from build123d import *

# Parameters (mm, degrees)
SALIENTE_EXTRUIR1_DEPTH = 1.6
CROQUIS3_R              = 4.2
SALIENTE_EXTRUIR2_DEPTH = 3
CROQUIS4_R              = 4.6
CORTAR_EXTRUIR1_DEPTH   = 1
CROQUIS5_R              = 3.5
CROQUIS5_R_2            = 3.45
SALIENTE_EXTRUIR3_DEPTH = 1
CROQUIS6_R              = 0.875
CORTAR_EXTRUIR2_DEPTH   = 22.438435028
CROQUIS7_R              = 1.4
CORTAR_EXTRUIR3_DEPTH   = 22.246329011
CROQUIS8_R              = 2.65
CORTAR_EXTRUIR4_DEPTH   = 3.4


with BuildPart() as part:
    # Croquis1 → Saliente-Extruir1 (new body)
    with BuildSketch(Plane(origin=(0, 0, 0), x_dir=(1, 0, 0), z_dir=(0, 1, 0))):
        with BuildLine():
            ThreePointArc((2.35, 13.321654392), (0, 15.671654392), (-2.35, 13.321654392))
            Line((-2.35, 13.321654392), (-3.5, 6.062177826))
            Line((-3.5, 6.062177826), (-10.361891124, 8.695986895))
            ThreePointArc((-10.361891124, 8.695986895), (-13.572050822, 7.835827196), (-12.711891124, 4.625667497))
            Line((-12.711891124, 4.625667497), (-7, 0))
            Line((-7, 0), (-12.711891124, -4.625667497))
            ThreePointArc((-12.711891124, -4.625667497), (-13.572050822, -7.835827196), (-10.361891124, -8.695986895))
            Line((-10.361891124, -8.695986895), (-3.5, -6.062177826))
            Line((-3.5, -6.062177826), (-2.35, -13.321654392))
            ThreePointArc((-2.35, -13.321654392), (0, -15.671654392), (2.35, -13.321654392))
            Line((2.35, -13.321654392), (3.5, -6.062177826))
            Line((3.5, -6.062177826), (10.361891124, -8.695986895))
            ThreePointArc((10.361891124, -8.695986895), (13.572050822, -7.835827196), (12.711891124, -4.625667497))
            Line((12.711891124, -4.625667497), (7, 0))
            Line((7, 0), (12.711891124, 4.625667497))
            ThreePointArc((12.711891124, 4.625667497), (13.572050822, 7.835827196), (10.361891124, 8.695986895))
            Line((10.361891124, 8.695986895), (3.5, 6.062177826))
            Line((3.5, 6.062177826), (2.35, 13.321654392))
        make_face()
    extrude(amount=SALIENTE_EXTRUIR1_DEPTH)

    # Croquis3 → Saliente-Extruir2 (add)
    with BuildSketch(Plane.XZ):
        with Locations(Location((0, 0, 0), (0, 0, 90))):
            Circle(CROQUIS3_R)
    extrude(amount=SALIENTE_EXTRUIR2_DEPTH)

    # Croquis4 → Cortar-Extruir1 (cut)
    with BuildSketch(Plane(origin=(0, 1.6, 0), x_dir=(1, 0, 0), z_dir=(0, 1, 0))):
        with Locations(Location((0, 0, 0), (0, 0, 270))):
            Circle(CROQUIS4_R)
    extrude(amount=-CORTAR_EXTRUIR1_DEPTH, mode=Mode.SUBTRACT)

    # Croquis5 → Saliente-Extruir3 (add)
    with BuildSketch(Plane(origin=(0, 0.6, 0), x_dir=(1, 0, 0), z_dir=(0, 1, 0))):
        with Locations(Location((0, 0, 0), (0, 0, 270))):
            Circle(CROQUIS5_R)
        with Locations(Location((0, 0, 0), (0, 0, 270))):
            Circle(CROQUIS5_R_2, mode=Mode.SUBTRACT)
    extrude(amount=SALIENTE_EXTRUIR3_DEPTH)

    # Croquis6 → Cortar-Extruir2 (cut, through all)
    with BuildSketch(Plane(origin=(0, 1.6, 0), x_dir=(1, 0, 0), z_dir=(0, 1, 0))):
        with Locations(Location((11.366583425, 6.5625, 0), (0, 0, 270))):
            Circle(CROQUIS6_R)
        with Locations(Location((9.114917375, 5.2625, 0), (0, 0, 270))):
            Circle(CROQUIS6_R)
        with Locations(Location((6.473539893, 3.7375, 0), (0, 0, 270))):
            Circle(CROQUIS6_R)
        with Locations(Location((11.366583425, -6.5625, 0), (0, 0, 270))):
            Circle(CROQUIS6_R)
        with Locations(Location((9.114917375, -5.2625, 0), (0, 0, 270))):
            Circle(CROQUIS6_R)
        with Locations(Location((6.473539893, -3.7375, 0), (0, 0, 270))):
            Circle(CROQUIS6_R)
        with Locations(Location((0, -13.125, 0), (0, 0, 270))):
            Circle(CROQUIS6_R)
        with Locations(Location((0, -10.525, 0), (0, 0, 270))):
            Circle(CROQUIS6_R)
        with Locations(Location((0, -7.475, 0), (0, 0, 270))):
            Circle(CROQUIS6_R)
        with Locations(Location((-11.366583425, -6.5625, 0), (0, 0, 270))):
            Circle(CROQUIS6_R)
        with Locations(Location((-9.114917375, -5.2625, 0), (0, 0, 270))):
            Circle(CROQUIS6_R)
        with Locations(Location((-6.473539893, -3.7375, 0), (0, 0, 270))):
            Circle(CROQUIS6_R)
        with Locations(Location((-11.366583425, 6.5625, 0), (0, 0, 270))):
            Circle(CROQUIS6_R)
        with Locations(Location((-9.114917375, 5.2625, 0), (0, 0, 270))):
            Circle(CROQUIS6_R)
        with Locations(Location((-6.473539893, 3.7375, 0), (0, 0, 270))):
            Circle(CROQUIS6_R)
        with Locations(Location((0, 13.125, 0), (0, 0, 270))):
            Circle(CROQUIS6_R)
        with Locations(Location((0, 10.525, 0), (0, 0, 270))):
            Circle(CROQUIS6_R)
        with Locations(Location((0, 7.475, 0), (0, 0, 270))):
            Circle(CROQUIS6_R)
    extrude(amount=-CORTAR_EXTRUIR2_DEPTH, mode=Mode.SUBTRACT)

    # Croquis7 → Cortar-Extruir3 (cut, through all)
    with BuildSketch(Plane(origin=(0, 0.6, 0), x_dir=(1, 0, 0), z_dir=(0, 1, 0))):
        with Locations(Location((0, 0, 0), (0, 0, 270))):
            Circle(CROQUIS7_R)
    extrude(amount=-CORTAR_EXTRUIR3_DEPTH, mode=Mode.SUBTRACT)

    # Croquis8 → Cortar-Extruir4 (cut)
    with BuildSketch(Plane.XZ.offset(3)):
        with Locations(Location((0, 0, 0), (0, 0, 270))):
            Circle(CROQUIS8_R)
    extrude(amount=-CORTAR_EXTRUIR4_DEPTH, mode=Mode.SUBTRACT)


solid = part.part
Source: CAD feature listing. Evaluate the final solid. Frame: model axes, mm. A direction names the side the tool comes from. Coordinates: 2 decimals unless noted, no trailing zeros. Order: outer loops, then holes, each group sorted by start corner. A loop starts at its lowest first (then second) coordinate and runs counter-clockwise, first axis right, second up.
Item 1: Cut plane D-D (x = 5). Return loops of the section in (y, z).
Output values:
outline: (0, -6.64) - (1.6, -6.64) - (1.6, 6.64) - (0, 6.64) - close
Item 2: First-contact query: P1, Ø1.6, axis at x = -6.47, z = -3.74, coming from the +Y side; P2, Ø2, axis at x = 6.47, z = 3.74, coming from the -Y side; P3, Ø1.5, axis at x = 1, y = -1, coming from the -Z side; P4, Ø5.5, axis at x = 0, z = 0, coming from the +Y side. Flat tips, straight axial feed; report the tip coordinate or a pass-through.
Output values:
P1: passes through
P2: stops at y = 0
P3: stops at z = -4.19
P4: stops at y = 0.6
Item 3: Material intervals for line 1 (Z direction, x = 9.5, y = 0.7); line 2 (Z direction, x = 6, y = 0.5); line 3 (Y direction, x = 2.5, z = -1), sorted ascending.
Output values:
line 1: z = -8.37 to -6.05, -4.48 to -2.02, 2.02 to 4.48, 6.05 to 8.37
line 2: z = -7.02 to -4.47, -3 to 3, 4.47 to 7.02
line 3: y = -3 to 0.6
Item 4: Set-up query: faces 4 (the face through (-0.05, 0.79, 15.67)), 5 (the face through (1.38, 1.11, 4.39)), 6 (the face through (-9.9, 0.79, -2.35)), 7 (the face through (6.98, 0.79, -7.4)), 8 (the face through (9.816, 0.789, -2.28)). Return all of +Z, -Z, +X, -X, +Y, -Y with unobstructed straight access to the full face (end or side cutting, diameter ignored); none if empty.
Output values:
face 4: +Z, +Y, -Y
face 5: +Y
face 6: -X, +Y, -Y
face 7: -Z, +Y, -Y
face 8: +X, +Y, -Y
Item 5: Pull-direction query (Z, two-part tool) for faces 1 (the face through (-2.933, 0.789, 9.641)), 2 (the face through (-5.606, 0.811, -3.851)), 3 (the face through (-2.917, 0.789, -9.743)); classes: pulls with the +Z half, pulls with the -Z half, needs draft (parallel to the pull), parting line crosses it, or undercut.
Output values:
face 1: pulls with the +Z half
face 2: undercut
face 3: pulls with the -Z half
Item 6: Cut plane B-B (y = -1.6). Return loops of the section in (x, z), plus the area to 3 significant figures.
Output values:
outline: circle Ø8.4 at (0, 0); hole circle Ø5.3 at (0, 0)
area: 33.4 mm2
Item 7: Cut plane A-A (x = 0). Count the separate pieces of the cut face and the enclosed holes in it, plus the area to 3 significant figures.
Output values:
separate pieces: 8
enclosed holes: 0
area: 30.9 mm2
